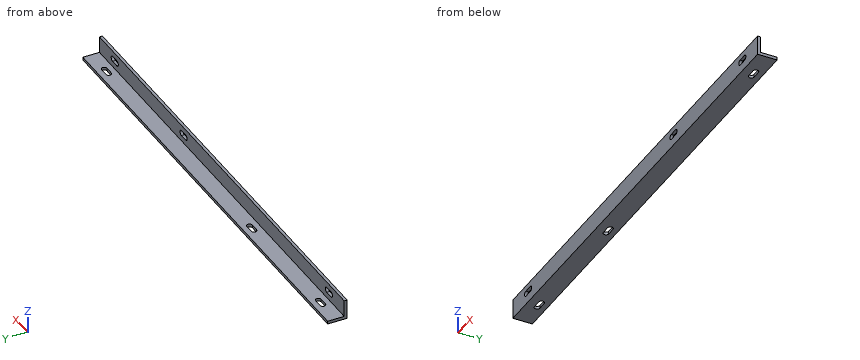
```python
from build123d import *

# Parameters (mm, degrees)
F1_DEPTH = 480
F3_DEPTH = 3
F5_DEPTH = 3


with BuildPart() as f1:
    # F0 (on Right) → F1 (new body)
    with BuildSketch(Plane.YZ):
        Polygon((0, 20), (0, 0), (20, 0), (20, 3), (3, 3), (3, 20), align=None)
    extrude(amount=F1_DEPTH)

    # F2 (on face) → F3 (cut)
    with BuildSketch(Plane(origin=(0, 3, 0), x_dir=(-1, 0, 0), z_dir=(0, 1, 0))):
        with BuildLine():
            Line((-445.75, 14.25), (-454.25, 14.25))
            ThreePointArc((-454.25, 14.25), (-457, 11.5), (-454.25, 8.75))
            Line((-454.25, 8.75), (-445.75, 8.75))
            ThreePointArc((-445.75, 8.75), (-443, 11.5), (-445.75, 14.25))
        make_face()
        with BuildLine():
            Line((-25.75, 14.25), (-34.25, 14.25))
            ThreePointArc((-34.25, 14.25), (-37, 11.5), (-34.25, 8.75))
            Line((-34.25, 8.75), (-25.75, 8.75))
            ThreePointArc((-25.75, 8.75), (-23, 11.5), (-25.75, 14.25))
        make_face()
        with BuildLine():
            Line((-310.75, 14.25), (-319.25, 14.25))
            ThreePointArc((-319.25, 14.25), (-322, 11.5), (-319.25, 8.75))
            Line((-319.25, 8.75), (-310.75, 8.75))
            ThreePointArc((-310.75, 8.75), (-308, 11.5), (-310.75, 14.25))
        make_face()
    extrude(amount=-F3_DEPTH, mode=Mode.SUBTRACT)

    # F4 (on face) → F5 (cut)
    with BuildSketch(Plane.XY.offset(3)):
        with BuildLine():
            Line((454.25, 14.25), (445.75, 14.25))
            ThreePointArc((445.75, 14.25), (443, 11.5), (445.75, 8.75))
            Line((445.75, 8.75), (454.25, 8.75))
            ThreePointArc((454.25, 8.75), (457, 11.5), (454.25, 14.25))
        make_face()
        with BuildLine():
            Line((169.25, 14.25), (160.75, 14.25))
            ThreePointArc((160.75, 14.25), (158, 11.5), (160.75, 8.75))
            Line((160.75, 8.75), (169.25, 8.75))
            ThreePointArc((169.25, 8.75), (172, 11.5), (169.25, 14.25))
        make_face()
        with BuildLine():
            Line((34.25, 14.25), (25.75, 14.25))
            ThreePointArc((25.75, 14.25), (23, 11.5), (25.75, 8.75))
            Line((25.75, 8.75), (34.25, 8.75))
            ThreePointArc((34.25, 8.75), (37, 11.5), (34.25, 14.25))
        make_face()
    extrude(amount=-F5_DEPTH, mode=Mode.SUBTRACT)


solid = f1.part
```
Model file for the job. Use its own axes, mm. Coordinates: 2 decimals unless noted, no trailing zeros. Write each loop counter-clockwise with the first axis right and the second up, starting at its lowest first coordinate (ties: lowest second). Pieces come first, ordered by that corner, then holes. Notation, with made-up numbers: (-19, 60.5) - (6, 60.5) arc R26 cw to (6, 93.5) - close; hole circle Ø4 at (53.25, 46). An arc over 180 degrees is marked (long way). Use a Markdown table: item, result. Add a question column.
Item 1: Drop flat-ended pins along their axis: pin 1 (1 mm diameter, centred on x = 248, y = 12, fed in from -Z); pin 2 (8 mm diameter, centred on x = 113, z = 8, fed in from +Y); pin 3 (8.5 mm diameter, centred on x = 145, y = 15.5, fed in from +Z). Give the stop position or say it passes through.
Item 2: Drill centre line: line 1 along Z through (x, y) = (27, 16.5). Where is it in solid material? Low to high.
Item 3: Band-saw the part on A-A, the plane x = 227.5. Write the cut outline in (y, z), and give its area (3 significant figures).
A:
| question | item | result |
|---|---|---|
| 1 | pin 1 | stops at z = 0 |
| 1 | pin 2 | stops at y = 3 |
| 1 | pin 3 | stops at z = 3 |
| 2 | line 1 | z = 0 to 3 |
| 3 | outline | (0, 0) - (20, 0) - (20, 3) - (3, 3) - (3, 20) - (0, 20) - close |
| 3 | area | 111 mm² |
